CAD build for the part. Positions are in the model's coordinates, mm. Face numbers are marked on the shaded views. A direction names the side the tool comes from. Give positions to 0.01 mm unless a question says otherwise; leave off trailing zeros. Order: outer loops, then holes, each group sorted by start corner. A loop starts at its lowest first (then second) coordinate and runs counter-clockwise, first axis right, second up. Notation, with made-up numbers: M -29.5,-30 L 16.5,-30 A21 cw 16.5,9 Z; hole C 65.5,57 d10. An arc over 180 degrees is marked long. Put each result on its own line as item: value. Start each with the question number.
1) Tool access for the marked faces 1, 2, 3, 4 and 5: list every direction of +Z, -Z, +X, -X, +Y, -Y with a clear straight run to the whole face (end or side of a thin tool).
2) Cut at D-D (y = -2). Write the cut outline in (x, z), and give its area (3 significant figures).
3) Two-plate mould, pull along X, no slides. Class the marked faces 6, 7 and 8: released by +X, released by -X, zero draft, split by the parting line, or undercut.
4) Cut at C-C (z = 0.5). Write the cut outline in (x, y).
5) Pin check, flat tips, straight feed: pin 1 (6 mm diameter, centred on x = 4.5, y = 6.5, fed in from -Z); pin 2 (1.9 mm diameter, centred on y = 1.5, z = 7.5, fed in from -X); pin 3 (5 mm diameter, centred on y = -3.5, z = 1.5, fed in from +X); pin 4 (1.6 mm diameter, centred on x = 0, z = 9, fed in from +Y). Stop position of each tip, or through.
6) Cut at A-A (z = 3.5). Write the cut outline in (x, y), and give its area (3 significant figures).
7) Cut at B-B (x = 0). Write the cut outline in (y, z).
8) Drill centre lines: line 1 (Z direction, x = 0, y = -7.25); line 2 (Z direction, x = 0, y = 6.75); line 3 (Y direction, x = 8.25, z = 4.75). Where is each one in solid material? Low to high. Write a range as [from, to].
Autodesk Inventor part; units mm, degrees
ref_plane "YZ Plane" through (0, 0, 0) normal (1, 0, 0) x (0, 1, 0)
ref_plane "XZ Plane" through (0, 0, 0) normal (0, 1, 0) x (-1, 0, 0)
ref_plane "XY Plane" through (0, 0, 0) normal (0, 0, 1) x (1, 0, 0)
sketch "Sketch1" plane through (0, 0, 0) normal (0, 0, 1) x (1, 0, 0)
  circle A0 centre (0, 0) radius 10
  dimension "d0" = 20
extrude "Extrusion1" add sketch "Sketch1" along normal blind 14.5
sketch "Sketch2" plane through (0, 0, 0) normal (0, 0, -1) x (-1, 0, 0)
  line L0 (-1.5, -2.5) -> (1.5, -2.5)
  line L1 (1.5, -2.5) -> (1.5, 2.5)
  line L2 (1.5, 2.5) -> (-1.5, 2.5)
  line L3 (-1.5, 2.5) -> (-1.5, -2.5)
  point P0 (0, 0)
  dimension "d3" = 3
  dimension "d4" = 5
  dimension "d5" = 2.5
  dimension "d6" = 1.5
extrude "Extrusion2" cut sketch "Sketch2" against normal blind 10
sketch "Sketch4" plane through (0, 0, 0) normal (0, 0, -1) x (-1, 0, 0)
  circle A0 centre (0, 0) radius 4.5
  dimension "d12" = 9
extrude "Extrusion4" [suppressed]
sketch "Sketch10" plane through (0, 0, 14.5) normal (0, 0, 1) x (1, 0, 0)
  line L0 (1.59, 2.754) -> (3.18, 0)
  line L1 (3.18, 0) -> (1.59, -2.754)
  line L2 (1.59, -2.754) -> (-1.59, -2.754)
  line L3 (-1.59, -2.754) -> (-3.18, 0)
  line L4 (-3.18, 0) -> (-1.59, 2.754)
  line L5 (-1.59, 2.754) -> (1.59, 2.754)
  point P0 (0, 0)
  point P1 (0, 0)
  dimension "d63" = 3.18
extrude "Extrusion7" cut sketch "Sketch10" against normal blind 9
ref_plane "Work Plane3" through (0, -10, 0) normal (0, -1, 0) x (1, 0, 0)
sketch "Sketch11" plane through (0, -10, 0) normal (0, -1, 0) x (1, 0, 0)
  circle A0 centre (0, 12) radius 1.45
  line L0 (10, 14.5) -> (-10, 14.5)
  point P0 (0, 0)
  dimension "d66" = 2.9
  dimension "d128" = 2.5
extrude "Extrusion8" cut sketch "Sketch11" against normal through all
ref_plane "Work Plane4" through (-10.5, -2.5, 0) normal (-1, 0, 0) x (0, 0, 1)
sketch "Sketch12" plane through (-10.5, -2.5, 0) normal (-1, 0, 0) x (0, 0, 1)
  circle A0 centre (3.5, 2.5) radius 1.45
  line L0 (0, 0) -> (5.5, 0)
  point P0 (0, 2.5)
  dimension "d71" = 2.9
  dimension "d74" = 3.5
  dimension "d124" = 2.5
extrude "Extrusion9" cut sketch "Sketch12" against normal blind 22
sketch "Sketch16" plane through (0, 0, 0) normal (0, 0, -1) x (-1, 0, 0)
  line L0 (-13.5, 7.2115) -> (-9.5, 7.2115)
  line L1 (-9.5, 7.2115) -> (-9.5, -8.6118)
  line L2 (-9.5, -8.6118) -> (-13.5, -8.6118)
  line L3 (-13.5, -8.6118) -> (-13.5, 7.2115)
  line L4 (9.5, 9.312) -> (14.5, 9.312)
  line L5 (14.5, 9.312) -> (14.5, -11.179)
  line L6 (14.5, -11.179) -> (9.5, -11.179)
  line L7 (9.5, -11.179) -> (9.5, 9.312)
  line L8 (-14.4464, 13.5) -> (12.1592, 13.5)
  line L9 (12.1592, 13.5) -> (12.1592, 9.5)
  line L10 (12.1592, 9.5) -> (-14.4464, 9.5)
  line L11 (-14.4464, 9.5) -> (-14.4464, 13.5)
  line L12 (-12.7193, -13.5) -> (12.1592, -13.5)
  line L13 (12.1592, -13.5) -> (12.1592, -9.5)
  line L14 (12.1592, -9.5) -> (-12.7193, -9.5)
  line L15 (-12.7193, -9.5) -> (-12.7193, -13.5)
  line L16 (1.5, -2.5) -> (-1.5, -2.5)
  line L17 (-1.5, -2.5) -> (-1.5, 2.5)
  line L18 (-1.5, 2.5) -> (1.5, 2.5)
  line L19 (1.5, 2.5) -> (1.5, -2.5)
  point P0 (-12.5, -8.5)
  point P1 (11.5, -8.5)
  point P2 (11.5, 8.5)
  point P3 (8.5, 8.5)
  point P4 (9.5, -9.5)
  point P5 (-8.5, -8.5)
  point P6 (12.1592, 9.312)
  point P7 (12.1592, -11.179)
  dimension "d104" = 4
  dimension "d105" = 7
  dimension "d106" = 8
  dimension "d107" = 7
  dimension "d108" = 8
  dimension "d109" = 5
  dimension "d110" = 4
  dimension "d111" = 4
extrude "Extrusion13" cut sketch "Sketch16" against normal through all contours L0 L1 L2 L3 | L4 L5 L6 L13 L14 L7 | L14 L13 L6 L7 | L7 L6 L13 L12 L15 L14 | L8 L9 L10 L11
sketch "Sketch18" plane through (0, 0, 0) normal (0, 0, -1) x (-1, 0, 0)
  circle A0 centre (0, 0) radius 12.5
  line L0 (-1.5, -2.5) -> (-1.5, 2.5)
  line L1 (1.5, 2.5) -> (1.5, -2.5)
  line L2 (-1.5, 2.5) -> (1.5, 2.5)
  line L3 (1.5, 2.5) -> (1.5, -2.5)
  line L4 (1.5, -2.5) -> (-1.5, -2.5)
  line L5 (-1.5, -2.5) -> (-1.5, 2.5)
  dimension "d118" = 25
extrude "Extrusion15" add sketch "Sketch18" along normal blind 3.8
chamfer "Chamfer1" distance 4.75 angle 45 4 edges at (1.5, 0, -3.8) (0, 2.5, -3.8) (0, -2.5, -3.8) (-1.5, 0, -3.8)
sketch "Sketch19" plane through (-9.5, -3.1225, 14.5) normal (-1, 0, 0) x (0, 0, 1)
  circle A0 centre (-11, 3.1225) radius 1.45
  circle A1 centre (-11, 3.1225) radius 4.5
  point P0 (-14.5, 3.1225)
  dimension "d125" = 9
extrude "Extrusion16" cut sketch "Sketch19" along normal blind 5 contours A0 | A1
equation "\"d107\" = d105"
equation "\"d108\" = d106"
properties part number "3mm_shaft_couple_sideclip_v3"
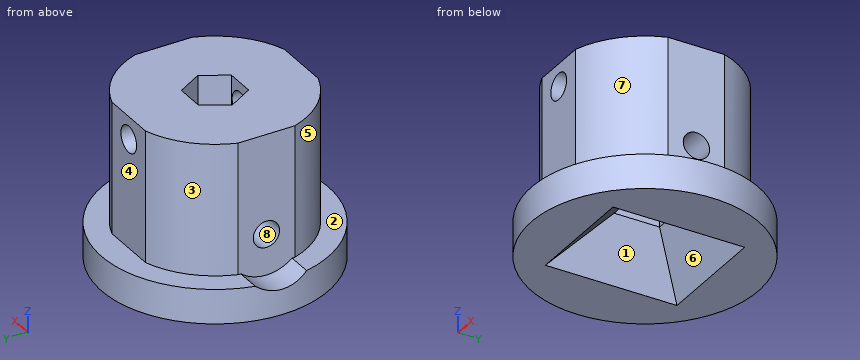
Solution:
1. face 1: -Z
1. face 2: +Z
1. face 3: +Z, -X, +Y
1. face 4: +Z, +X, -X, +Y
1. face 5: +Z, -X, -Y
2. outline: M -12.34,-3.8 L -6.25,-3.8 L -1.5,0.95 L -1.5,5.5 L -2.03,5.5 L -2.03,14.5 L -9.5,14.5 L -9.5,-0.53 L -12.34,-0.53 Z; M 1.5,0.95 L 6.25,-3.8 L 12.34,-3.8 L 12.34,0 L 9.5,0 L 9.5,14.5 L 2.03,14.5 L 2.03,5.5 L 1.5,5.5 Z
2. area: 281 mm²
3. face 6: undercut
3. face 7: released by +X
3. face 8: zero draft
4. outline: M -9.5,-3.12 A10 ccw -3.12,-9.5 L 3.12,-9.5 A10 ccw 9.5,-3.12 L 9.5,3.12 A10 ccw 3.12,9.5 L -3.12,9.5 A10 ccw -9.5,3.12 Z; hole M -1.95,-2.95 L 1.95,-2.95 L 1.95,2.95 L -1.95,2.95 Z
5. pin 1: z = -3.8
5. pin 2: x = -9.5
5. pin 3: x = 12.41
5. pin 4: y = 9.5
6. outline: M -9.5,-3.12 A10 ccw -3.12,-9.5 L 3.12,-9.5 A10 ccw 9.5,-3.12 L 9.5,-1.45 L 1.5,-1.45 L 1.5,-2.5 L -1.5,-2.5 L -1.5,-1.45 L -9.5,-1.45 Z; M -9.5,1.45 L -1.5,1.45 L -1.5,2.5 L 1.5,2.5 L 1.5,1.45 L 9.5,1.45 L 9.5,3.12 A10 ccw 3.12,9.5 L -3.12,9.5 A10 ccw -9.5,3.12 Z
6. area: 244 mm²
7. outline: M -12.5,-3.8 L -7.25,-3.8 L -2.5,0.95 L -2.5,5.5 L -2.75,5.5 L -2.75,10.55 L -9.5,10.55 L -9.5,0 L -12.5,0 Z; M -9.5,13.45 L -2.75,13.45 L -2.75,14.5 L -9.5,14.5 Z; M 2.5,0.95 L 7.25,-3.8 L 12.5,-3.8 L 12.5,0 L 9.5,0 L 9.5,10.55 L 2.75,10.55 L 2.75,5.5 L 2.5,5.5 Z; M 2.75,13.45 L 9.5,13.45 L 9.5,14.5 L 2.75,14.5 Z
8. line 1: [-3.8, 10.55], [13.45, 14.5]
8. line 2: [-3.3, 10.55], [13.45, 14.5]
8. line 3: [-5.65, -0.73], [0.73, 5.65]
